Autodesk Inventor part; units mm, degrees
ref_plane "YZ Plane" through (0, 0, 0) normal (1, 0, 0) x (0, 1, 0)
ref_plane "XZ Plane" through (0, 0, 0) normal (0, 1, 0) x (-1, 0, 0)
ref_plane "XY Plane" through (0, 0, 0) normal (0, 0, 1) x (1, 0, 0)
sketch "Sketch1" plane through (0, 0, 0) normal (0, 0, 1) x (1, 0, 0)
  line L0 (6.8, 0) -> (8.075, 0)
  line L1 (12.75, -2.6991) -> (12.75, -5.8)
  line L2 (7.75, -6.4) -> (5, -6.4)
  line L3 (5, -6.4) -> (5, -26.4)
  line L4 (5, -26.4) -> (0, -26.4)
  line L5 (0, -26.4) -> (0, 0)
  line L6 (7.75, -6.4) -> (7.75, -5.8)
  line L7 (7.75, -5.8) -> (12.75, -5.8)
  line L8 (0, -1.28) -> (6.5, -1.28)
  line L9 (6.8, -0.98) -> (6.8, 0)
  line L10 (8.075, 0) -> (12.75, -2.6991)
  arc A0 (6.5, -1.28) -> (6.8, -0.98) centre (6.5, -0.98) ccw
  dimension "d0" = 25.5
  dimension "d1" = 10
  dimension "d3" = 20
  dimension "d4" = 15.5
  dimension "d5" = 0.6
  dimension "d26" = 16.15
  dimension "d27" = 30
  dimension "d28" = 13.6
  dimension "d29" = 1.28
  dimension "d30" = 0.3
  dimension "d31" = 6.4
revolve "Revolution1" add sketch "Sketch1" angle 360 about axis through (0, -26.4, 0) along (0, 1, 0)
sketch "Sketch2" plane through (0, 0, 0) normal (0, 1, 0) x (1, 0, 0)
  line L0 (0, -9.815) -> (-8.5, -4.9075)
  line L1 (-8.5, -4.9075) -> (-8.5, 4.9075)
  line L2 (-8.5, 4.9075) -> (0, 9.815)
  line L3 (0, 9.815) -> (8.5, 4.9075)
  line L4 (8.5, 4.9075) -> (8.5, -4.9075)
  line L5 (8.5, -4.9075) -> (0, -9.815)
  circle A0 centre (0, 0) radius 12.75
  point P0 (0, 0)
  point P1 (0, 0)
  dimension "d32" = 17
extrude "Extrusion1" cut sketch "Sketch2" against normal blind 5.8
thread "Thread1"
chamfer "Chamfer1" distance 0.8333 angle 45 1 edges at (-5, -26.4, 0)
equation "\"d0\" = 1.5 * S_"
equation "\"d1\" = d1_"
equation "\"d3\" = L"
equation "\"d4\" = dw"
equation "\"d5\" = hw"
equation "\"d26\" = 0.95 * S_"
equation "\"d28\" = 0.8 * S_"
equation "\"d29\" = 0.2 * k"
equation "\"d31\" = k"
equation "\"d14\" = b"
equation "\"d16\" = 0.0833333 * d"
equation "\"d32\" = S_"
equation "\"d33\" = k - hw"
equation "\"d1_\" = 10"
equation "\"S_\" = 17"
equation "\"k\" = 6.4"
equation "\"e\" = 18.7"
equation "\"L\" = 20"
equation "\"b\" = 18"
equation "\"Grip_Length\" = 2"
equation "\"dw\" = 15.5"
equation "\"hw\" = 0.6"
properties part number "Bolt 4A M10-6g×20 GOST 7798-70" material "Steel, Mild"
Here's how the part is built. I have some questions about the finished solid (model axes, mm). A direction names the side the tool comes from. Give positions to 0.01 mm unless a question says otherwise; leave off trailing zeros. Order: outer loops, then holes, each group sorted by start corner. A loop starts at its lowest first (then second) coordinate and runs counter-clockwise, first axis right, second up. Notation, with made-up numbers: (69, -22.5) -> (120, -22.5) arc R28 cw to (120, 13.5) -> close; hole circle Ø1 at (31.25, 40.5). An arc over 180 degrees is marked (long way). One line per item, written item: value. Start each with the question number.
1. Imagine slicing it at A-A, the plane z = 0. List the corners of the cut face in (x, y) for me (3 decimals), plus the area to 3 significant figures.
2. Imagine slicing it at B-B, the plane y = -19.25. List the corners of the cut face in (x, z) for me, plus the area to 3 significant figures.
3. For faces 1 (the face through (-1.009, -6.096, -7.684)), 2 (the face through (0, -26.4, 0)), which set-ups out of +Z, -Z, +X, -X, +Y, -Y let a thin tool reach every point of the face, with its end or its side?
4. Imagine slicing it at C-C, the plane y = -4. List the corners of the cut face in (x, z) for me (1 decimal).
5. Will these pins go through, and if not, where does the flat tip stop? pin 1 Ø1 at (x, z) = (-2.5, 8) entering from +Y; pin 2 Ø10 at (x, y) = (0.5, -14) entering from +Z; pin 3 Ø8 at (x, y) = (-5.5, -21.5) entering from -Z; pin 4 Ø10 at (x, z) = (-6.5, -6.5) entering from -Y.
6. I need wall thicknesses on probe 1 along X at (y, z) = (-0.7, 0); probe 2 along Y at (x, z) = (1.25, -6.25); probe 3 along X at (y, z) = (-22.25, 0). Which ranges of each line are inside material? Lowest first, please. Write a range as from..to.
7. We'd pull the mould along Z, two halves only. Please class faces 3 (the face through (-1.47, -0.48, 6.64)), 4 (the face through (0, -1.28, 0)), 5 (the face through (-4, 0, 6)), 6 (the face through (4.19, -2.984, -7.396)): released by +Z, released by -Z, zero draft, split by the parting line, or undercut.
Values follow:
1. outline: (-8.5, -5.8) -> (-7.75, -5.8) -> (-7.75, -6.4) -> (-5, -6.4) -> (-5, -25.567) -> (-4.167, -26.4) -> (4.167, -26.4) -> (5, -25.567) -> (5, -6.4) -> (7.75, -6.4) -> (7.75, -5.8) -> (8.5, -5.8) -> (8.5, -0.245) -> (8.075, 0) -> (6.8, 0) -> (6.8, -0.98) arc R0.3 cw to (6.5, -1.28) -> (-6.5, -1.28) arc R0.3 cw to (-6.8, -0.98) -> (-6.8, 0) -> (-8.075, 0) -> (-8.5, -0.245) -> close
1. area: 290 mm2
2. outline: circle Ø10 at (0, 0)
2. area: 78.5 mm2
3. face 1: -Y
3. face 2: +Z, -Z, +X, -X, -Y
4. outline: (-8.5, -4.9) -> (0, -9.8) -> (8.5, -4.9) -> (8.5, 4.9) -> (0, 9.8) -> (-8.5, 4.9) -> close
5. pin 1: stops at y = 0
5. pin 2: stops at z = 5
5. pin 3: stops at z = -4.77
5. pin 4: stops at y = -26.37
6. probe 1: x = -8.5..-6.8, 6.8..8.5
6. probe 2: y = -6.4..-1.28
6. probe 3: x = -5..5
7. face 3: undercut
7. face 4: undercut
7. face 5: zero draft
7. face 6: released by -Z
